The model under review builds one solid part; all positions refer to its coordinate system, in mm. A direction names the side the tool comes from. Coordinates: 2 decimals unless noted, no trailing zeros. Order: outer loops, then holes, each group sorted by start corner. A loop starts at its lowest first (then second) coordinate and runs counter-clockwise, first axis right, second up. Notation, with made-up numbers: (59, 37.5) -> (83, 37.5) arc R9 ccw to (83, 49.5) -> close; hole circle Ø5 at (48, 71). An arc over 180 degrees is marked (long way). Use one line per item in the form item = value.
from build123d import *

# Parameters (mm, degrees)
BOSS_EXTRUDE1_DEPTH = 5
SKETCH2_R           = 1.05
CUT_EXTRUDE1_DEPTH  = 5
SKETCH3_R           = 2
CUT_EXTRUDE2_DEPTH  = 3
CUT_EXTRUDE3_DEPTH  = 69.419660917
SKETCH5_R           = 2.5
CUT_EXTRUDE5_DEPTH  = 69.419660917
CUT_EXTRUDE7_DEPTH  = 3


with BuildPart() as part:
    # Sketch1 → Boss-Extrude1 (new body)
    with BuildSketch(Plane(origin=(0, 0, 0), x_dir=(1, 0, 0), z_dir=(0, 1, 0))):
        with BuildLine():
            Line((-27.5, 60), (27.5, 60))
            ThreePointArc((27.5, 60), (31.035533906, 58.535533906), (32.5, 55))
            Line((32.5, 55), (32.5, -55))
            ThreePointArc((32.5, -55), (31.035533906, -58.535533906), (27.5, -60))
            Line((27.5, -60), (-27.5, -60))
            ThreePointArc((-27.5, -60), (-31.035533906, -58.535533906), (-32.5, -55))
            Line((-32.5, -55), (-32.5, 55))
            ThreePointArc((-32.5, 55), (-31.035533906, 58.535533906), (-27.5, 60))
        make_face()
    extrude(amount=BOSS_EXTRUDE1_DEPTH)

    # Sketch2 → Cut-Extrude1 (cut)
    with BuildSketch(Plane(origin=(0, 5, 0), x_dir=(1, 0, 0), z_dir=(0, 1, 0))):
        with Locations(Location((-28.5, 56, 0), (0, 0, 270))):
            Circle(SKETCH2_R)
        with Locations(Location((28.5, 56, 0), (0, 0, 270))):
            Circle(SKETCH2_R)
        with Locations(Location((28.5, -56, 0), (0, 0, 270))):
            Circle(SKETCH2_R)
        with Locations(Location((-28.5, -56, 0), (0, 0, 270))):
            Circle(SKETCH2_R)
    extrude(amount=-CUT_EXTRUDE1_DEPTH, mode=Mode.SUBTRACT)

    # Sketch3 → Cut-Extrude2 (cut)
    with BuildSketch(Plane(origin=(0, 5, 0), x_dir=(1, 0, 0), z_dir=(0, 1, 0))):
        with Locations(Location((-28.5, 56, 0), (0, 0, 270))):
            Circle(SKETCH3_R)
        with Locations(Location((28.5, 56, 0), (0, 0, 270))):
            Circle(SKETCH3_R)
        with Locations(Location((28.5, -56, 0), (0, 0, 270))):
            Circle(SKETCH3_R)
        with Locations(Location((-28.5, -56, 0), (0, 0, 270))):
            Circle(SKETCH3_R)
    extrude(amount=-CUT_EXTRUDE2_DEPTH, mode=Mode.SUBTRACT)

    # Sketch4 → Cut-Extrude3 (cut, through all)
    with BuildSketch(Plane(origin=(0, 5, 0), x_dir=(1, 0, 0), z_dir=(0, 1, 0))):
        with BuildLine():
            ThreePointArc((7, 30.254330519), (4.949747468, 35.204077987), (0, 37.254330519))
            Line((0, 37.254330519), (0, 23.254330519))
            ThreePointArc((0, 23.254330519), (4.949747468, 25.304583051), (7, 30.254330519))
        make_face()
        with BuildLine():
            Line((0, 23.254330519), (0, 37.254330519))
            ThreePointArc((0, 37.254330519), (-7, 30.254330519), (0, 23.254330519))
        make_face()
    extrude(amount=-CUT_EXTRUDE3_DEPTH, mode=Mode.SUBTRACT)

    # Sketch5 → Cut-Extrude5 (cut, through all)
    with BuildSketch(Plane(origin=(0, 5, 0), x_dir=(1, 0, 0), z_dir=(0, 1, 0))):
        with Locations(Location((22.5, 50, 0), (0, 0, 270))):
            Circle(SKETCH5_R)
        with Locations(Location((0, -3.584481164, 0), (0, 0, 270))):
            Circle(SKETCH5_R)
        with Locations(Location((11.568109832, -18.584481164, 0), (0, 0, 270))):
            Circle(SKETCH5_R)
        with Locations(Location((11.487471201, -41.402489438, 0), (0, 0, 270))):
            Circle(SKETCH5_R)
        with Locations(Location((-11.406832571, -41.406832571, 0), (0, 0, 270))):
            Circle(SKETCH5_R)
        with Locations(Location((-11.24555531, -18.584481164, 0), (0, 0, 270))):
            Circle(SKETCH5_R)
    extrude(amount=-CUT_EXTRUDE5_DEPTH, mode=Mode.SUBTRACT)

    # Sketch6 → Cut-Extrude7 (cut)
    with BuildSketch(Plane(origin=(0, 5, 0), x_dir=(1, 0, 0), z_dir=(0, 1, 0))):
        with BuildLine():
            Line((7.568109832, -13.584481164), (15.568109832, -13.584481164))
            ThreePointArc((15.568109832, -13.584481164), (16.275216613, -13.877374383), (16.568109832, -14.584481164))
            Line((16.568109832, -14.584481164), (16.568109832, -22.584481164))
            ThreePointArc((16.568109832, -22.584481164), (16.275216613, -23.291587945), (15.568109832, -23.584481164))
            Line((15.568109832, -23.584481164), (7.568109832, -23.584481164))
            ThreePointArc((7.568109832, -23.584481164), (6.86100305, -23.291587945), (6.568109832, -22.584481164))
            Line((6.568109832, -22.584481164), (6.568109832, -14.584481164))
            ThreePointArc((6.568109832, -14.584481164), (6.86100305, -13.877374383), (7.568109832, -13.584481164))
        make_face()
        with BuildLine():
            Line((-15.24555531, -13.584481164), (-7.24555531, -13.584481164))
            ThreePointArc((-7.24555531, -13.584481164), (-6.538448529, -13.877374383), (-6.24555531, -14.584481164))
            Line((-6.24555531, -14.584481164), (-6.24555531, -22.584481164))
            ThreePointArc((-6.24555531, -22.584481164), (-6.538448529, -23.291587945), (-7.24555531, -23.584481164))
            Line((-7.24555531, -23.584481164), (-15.24555531, -23.584481164))
            ThreePointArc((-15.24555531, -23.584481164), (-15.952662092, -23.291587945), (-16.24555531, -22.584481164))
            Line((-16.24555531, -22.584481164), (-16.24555531, -14.584481164))
            ThreePointArc((-16.24555531, -14.584481164), (-15.952662092, -13.877374383), (-15.24555531, -13.584481164))
        make_face()
        with BuildLine():
            Line((-15.406832571, -36.406832571), (-7.406832571, -36.406832571))
            ThreePointArc((-7.406832571, -36.406832571), (-6.69972579, -36.69972579), (-6.406832571, -37.406832571))
            Line((-6.406832571, -37.406832571), (-6.406832571, -45.406832571))
            ThreePointArc((-6.406832571, -45.406832571), (-6.69972579, -46.113939352), (-7.406832571, -46.406832571))
            Line((-7.406832571, -46.406832571), (-15.406832571, -46.406832571))
            ThreePointArc((-15.406832571, -46.406832571), (-16.113939352, -46.113939352), (-16.406832571, -45.406832571))
            Line((-16.406832571, -45.406832571), (-16.406832571, -37.406832571))
            ThreePointArc((-16.406832571, -37.406832571), (-16.113939352, -36.69972579), (-15.406832571, -36.406832571))
        make_face()
        with BuildLine():
            Line((7.487471201, -36.402489438), (15.487471201, -36.402489438))
            ThreePointArc((15.487471201, -36.402489438), (16.194577983, -36.695382657), (16.487471201, -37.402489438))
            Line((16.487471201, -37.402489438), (16.487471201, -45.402489438))
            ThreePointArc((16.487471201, -45.402489438), (16.194577983, -46.10959622), (15.487471201, -46.402489438))
            Line((15.487471201, -46.402489438), (7.487471201, -46.402489438))
            ThreePointArc((7.487471201, -46.402489438), (6.78036442, -46.10959622), (6.487471201, -45.402489438))
            Line((6.487471201, -45.402489438), (6.487471201, -37.402489438))
            ThreePointArc((6.487471201, -37.402489438), (6.78036442, -36.695382657), (7.487471201, -36.402489438))
        make_face()
        with BuildLine():
            Line((-4, 1.415518836), (4, 1.415518836))
            ThreePointArc((4, 1.415518836), (4.707106781, 1.122625617), (5, 0.415518836))
            Line((5, 0.415518836), (5, -7.584481164))
            ThreePointArc((5, -7.584481164), (4.707106781, -8.291587945), (4, -8.584481164))
            Line((4, -8.584481164), (-4, -8.584481164))
            ThreePointArc((-4, -8.584481164), (-4.707106781, -8.291587945), (-5, -7.584481164))
            Line((-5, -7.584481164), (-5, 0.415518836))
            ThreePointArc((-5, 0.415518836), (-4.707106781, 1.122625617), (-4, 1.415518836))
        make_face()
    extrude(amount=-CUT_EXTRUDE7_DEPTH, mode=Mode.SUBTRACT)


solid = part.part
Item 1: To check wall thickness, follow L1, parallel to Z at x = 8, y = 3.7; L2, parallel to Z at x = 11.5, y = 0.75; L3, parallel to X at y = 2.8, z = 20. State the ranges of each line that lie inside material, in increasing order. Write a range as from..to.
Results found:
L1 = -60..13.58, 23.58..36.4, 46.4..60
L2 = -60..16.09, 21.08..38.9, 43.9..60
L3 = -32.5..-16.25, -6.25..6.57, 16.57..32.5
Item 2: We need section B-B (x = 22.5). Write out the cut boundary in (y, z), plus the area to 3 significant figures.
Results found:
outline = (0, -60) -> (5, -60) -> (5, -52.5) -> (0, -52.5) -> close; (0, -47.5) -> (5, -47.5) -> (5, 60) -> (0, 60) -> close
area = 575 mm²
Item 3: Clearance check with a flat-ended pin moving along its axis: pin 1 (6.5 mm diameter, centred on x = -11.41, z = 41.41, fed in from +Y). State where the tip first meets the part, or that it passes through.
Results found:
pin_1 = 2
Item 4: Tool access review of faces 1 (the face through (-32.5, 2, 1)), 2 (the face through (5, 4, 4)): name each direction out of +Z, -Z, +X, -X, +Y, -Y from which nothing blocks a thin tool from reaching the whole face with its end or side.
Results found:
face_1 = +Z, -Z, -X, +Y, -Y
face_2 = +Y
Item 5: We need section D-D (y = 3.05). State how many separate pieces and enclosed holes the cut face has, plus the area to 3 significant figures.
Results found:
separate_pieces = 1
enclosed_holes = 11
area = 7,060 mm²
Item 6: Draft analysis for pull direction Z (two halves, no side actions). For faces 3 (the face through (8, 5, -1)), 4 (the face through (-6.246, 4, 19)), 5 (the face through (-11, 4, 13.584)), 6 (the face through (31, 2.46, -58.57)), state which applies: released by +Z, released by -Z, zero draft, split by the parting line, or undercut.
Results found:
face_3 = zero draft
face_4 = undercut
face_5 = undercut
face_6 = released by -Z
Item 7: We need section C-C (z = 18.5). Write out the cut boundary in (x, y).
Results found:
outline = (-32.5, 0) -> (-13.74, 0) -> (-13.74, 2) -> (-16.25, 2) -> (-16.25, 5) -> (-32.5, 5) -> close; (-8.75, 0) -> (9.07, 0) -> (9.07, 2) -> (6.57, 2) -> (6.57, 5) -> (-6.25, 5) -> (-6.25, 2) -> (-8.75, 2) -> close; (14.07, 0) -> (32.5, 0) -> (32.5, 5) -> (16.57, 5) -> (16.57, 2) -> (14.07, 2) -> close
Item 8: We need section A-A (z = -50). Write out the cut boundary in (x, y).
Results found:
outline = (-32.5, 0) -> (20, 0) -> (20, 5) -> (-32.5, 5) -> close; (25, 0) -> (32.5, 0) -> (32.5, 5) -> (25, 5) -> close
